from build123d import *

# Parameters (mm, degrees)
SKETCH1_R                  = 35
SKETCH1_R_2                = 6
SKETCH1_R_3                = 5
SKETCH1_W                  = 50
SKETCH1_H                  = 25
BOSS_EXTRUDE2_DEPTH        = 5.588
F_4_7_4_7_DIAMETER_HOLE1_D = 4.7
FILLET1_R                  = 1
FILLET2_R                  = 1
FILLET6_R                  = 4
FILLET7_R                  = 4
FILLET8_R                  = 4
FILLET9_R                  = 2
FILLET10_R                 = 2


with BuildPart() as part:
    # Sketch1 → Boss-Extrude2 (new body)
    with BuildSketch(Plane(origin=(0, 0, 0), x_dir=(1, 0, 0), z_dir=(0, 1, 0))):
        with Locations((32.785, 18.724314586)):
            Circle(SKETCH1_R)
        with Locations((32.785, 18.724314586)):
            Circle(SKETCH1_R_2, mode=Mode.SUBTRACT)
        with Locations((65.57, 0)):
            Circle(SKETCH1_R_3)
        Circle(SKETCH1_R_3)
        with Locations((32.785, 65.782929207)):
            Circle(SKETCH1_R_3)
        with Locations((32.785, 53.282929207)):
            Rectangle(SKETCH1_W, SKETCH1_H)
    extrude(amount=BOSS_EXTRUDE2_DEPTH)

    # Ø4.7 (4.7) Diameter Hole1 (through all)
    with Locations(Plane(origin=(0, 5.588, 0), x_dir=(1, 0, 0), z_dir=(0, 1, 0))):
        with Locations((0, 0), (65.57, 0), (32.785, 65.782929207)):
            Hole(F_4_7_4_7_DIAMETER_HOLE1_D / 2)

    # Fillet1
    fillet1_edges = [part.edges().sort_by_distance(p)[0] for p in [
        (27.785, 2.794, -65.782929207),
    ]]
    fillet(fillet1_edges, radius=FILLET1_R)

    # Fillet2
    fillet2_edges = [part.edges().sort_by_distance(p)[0] for p in [
        (37.785, 2.794, -65.782929207),
    ]]
    fillet(fillet2_edges, radius=FILLET2_R)

    # Fillet6
    fillet6_edges = [part.edges().sort_by_distance(p)[0] for p in [
        (0.603671593, 2.794, -4.963424282),
    ]]
    fillet(fillet6_edges, radius=FILLET6_R)

    # Fillet7
    fillet7_edges = [part.edges().sort_by_distance(p)[0] for p in [
        (4.581742742, 2.794, 2.001907453),
    ]]
    fillet(fillet7_edges, radius=FILLET7_R)

    # Fillet8
    fillet8_edges = [part.edges().sort_by_distance(p)[0] for p in [
        (60.988257258, 2.794, 2.001907453),
        (64.966328407, 2.794, -4.963424282),
    ]]
    fillet(fillet8_edges, radius=FILLET8_R)

    # Fillet9
    fillet9_edges = [part.edges().sort_by_distance(p)[0] for p in [
        (57.785, 2.794, -43.219212014),
    ]]
    fillet(fillet9_edges, radius=FILLET9_R)

    # Fillet10
    fillet10_edges = [part.edges().sort_by_distance(p)[0] for p in [
        (7.785, 2.794, -43.219212014),
    ]]
    fillet(fillet10_edges, radius=FILLET10_R)


solid = part.part
Input: part model. Units: mm. Frame: model coordinates. A direction names the side the tool comes from. Round coordinates to 2 decimals unless told otherwise and drop trailing zeros. Write each loop counter-clockwise with the first axis right and the second up, starting at its lowest first coordinate (ties: lowest second). Pieces come first, ordered by that corner, then holes.
1) Cut plane C-C (z = -23). Return the cut outline in (x, y).
2) Cut plane A-A (z = 0). Return the cut outline in (x, y).
3) Reachability of faces 4 (the flat face through (32, 0, -28)), 5 (the flat face through (57.785, 3, -55)), 6 (the flat face through (17, 3, -65.783)) from +Z, -Z, +X, -X, +Y, -Y: full face, straight path, thin tool, end or side. Return the list, or none.
4) Cut plane B-B (x = 33). Return the cut outline in (y, z), then the cut area to 3 significant figures.
5) Cut plane D-D (y = 2.8). Count the separate pieces of the cut face and the enclosed holes in it, then the cut area to 3 significant figures.
6) Ray query, L1, parallel to X at y = 2.3, z = -2; L2, parallel to X at y = 4.55, z = -1.5; L3, parallel to X at y = 4.1, z = -59 (3 decimals). Return the intervals inside material, ascending.
7) Contact query for flat-ended pins moving along their axis: P1, Ø1.7, axis at x = 49, y = 3, coming from the -Z side; P2, Ø3, axis at y = 2.5, z = -53.5, coming from the -X side (3 decimals); P3, Ø2, axis at y = 1.5, z = -50.5, coming from the +X side (3 decimals). Output: stop coordinate, or through.
8) Draft query along X for faces 1 (the cylindrical face through (-1.2, 2.8, -27.1)), 2 (the cylindrical face through (26.79, 2.75, -18.99)), 3 (the cylindrical face through (32.384, 2.755, 16.273)). Return one class per face: pulls with the +X half, pulls with the -X half, needs draft (parallel to the pull), parting line crosses it, or undercut.
Geometry says:
1. outline: (-1.95, 0) - (28.58, 0) - (28.58, 5.59) - (-1.95, 5.59) - close; (36.99, 0) - (67.52, 0) - (67.52, 5.59) - (36.99, 5.59) - close
2. outline: (-5, 0) - (-2.35, 0) - (-2.35, 5.59) - (-5, 5.59) - close; (2.35, 0) - (63.22, 0) - (63.22, 5.59) - (2.35, 5.59) - close; (67.92, 0) - (70.57, 0) - (70.57, 5.59) - (67.92, 5.59) - close
3. face 4: +Z, -Z, +X, -X, -Y
3. face 5: -Z, +X, +Y, -Y
3. face 6: -Z, -X, +Y, -Y
4. outline: (0, -70.78) - (5.59, -70.78) - (5.59, -68.12) - (0, -68.12) - close; (0, -63.44) - (5.59, -63.44) - (5.59, -24.72) - (0, -24.72) - close; (0, -12.73) - (5.59, -12.73) - (5.59, 16.28) - (0, 16.28) - close
4. area: 393 mm2
5. separate pieces: 1
5. enclosed holes: 4
5. area: 4,630 mm2
6. L1: x = -4.58 to -1.23, 1.23 to 64.34, 66.8 to 70.15
6. L2: x = -4.77 to -1.81, 1.81 to 63.76, 67.38 to 70.34
6. L3: x = 7.785 to 57.785
7. P1: stops at z = -65.78
7. P2: stops at x = 7.785
7. P3: stops at x = 57.785
8. face 1: pulls with the -X half
8. face 2: undercut
8. face 3: parting line crosses it
